Input: part model. Units: mm. Frame: model coordinates. Face numbers are marked on the shaded views. A direction names the side the tool comes from. Give positions to 0.01 mm unless a question says otherwise; leave off trailing zeros. Order: outer loops, then holes, each group sorted by start corner. A loop starts at its lowest first (then second) coordinate and runs counter-clockwise, first axis right, second up. Notation, with made-up numbers: (-12, -39.75) - (47, -39.75) arc R20 ccw to (47, -0.75) - close; hole circle Ø8 at (-28.5, 28). An arc over 180 degrees is marked (long way). Answer in a Markdown table with one row per item. Add a question column.
from build123d import *

# Parameters (mm, degrees)
BOSS_EXTRUDE3_DEPTH      = 1.5875
BOSS_EXTRUDE3_DEPTH_BACK = 43.175
SKETCH4_W                = 26.136325312
SKETCH4_H                = 38.4125
CUT_EXTRUDE1_DEPTH       = 14.701439982
SKETCH5_W                = 2
SKETCH5_H                = 2
BOSS_EXTRUDE5_DEPTH      = 44.7625
BOSS_EXTRUDE6_START      = -41.5875
SKETCH5_4_W              = 2
SKETCH5_4_H              = 2
BOSS_EXTRUDE6_DEPTH      = 38.4125


with BuildPart() as part:
    # Sketch3 → Boss-Extrude3 (new, two sides: drawn at the far end of the back side and taken through both)
    with BuildSketch(Plane.XY.offset(336.564940884).offset(-BOSS_EXTRUDE3_DEPTH_BACK)):
        with BuildLine():
            Line((-13.068162656, -2.834098381), (13.068162656, -2.834098381))
            ThreePointArc((13.068162656, -2.834098381), (15.189482999, -1.955418725), (16.068162656, 0.165901619))
            Line((16.068162656, 0.165901619), (16.068162656, 13.867341601))
            ThreePointArc((16.068162656, 13.867341601), (15.189482999, 15.988661944), (13.068162656, 16.867341601))
            Line((13.068162656, 16.867341601), (-13.068162656, 16.867341601))
            ThreePointArc((-13.068162656, 16.867341601), (-15.189482999, 15.988661944), (-16.068162656, 13.867341601))
            Line((-16.068162656, 13.867341601), (-16.068162656, 0.165901619))
            ThreePointArc((-16.068162656, 0.165901619), (-15.189482999, -1.955418725), (-13.068162656, -2.834098381))
        make_face()
    extrude(amount=BOSS_EXTRUDE3_DEPTH + BOSS_EXTRUDE3_DEPTH_BACK)

    # Sketch4 → Cut-Extrude1 (cut)
    with BuildSketch(Plane(origin=(0, 16.867341601, 0), x_dir=(1, 0, 0), z_dir=(0, 1, 0))):
        with Locations((0, -315.771190884)):
            Rectangle(SKETCH4_W, SKETCH4_H)
    extrude(amount=-CUT_EXTRUDE1_DEPTH, mode=Mode.SUBTRACT)

    # Sketch5 → Boss-Extrude5 (add)
    with BuildSketch(Plane.XY.offset(338.152440884)):
        with Locations((-17.068162656, 5)):
            Rectangle(SKETCH5_W, SKETCH5_H)
        with Locations((17.068162656, 5)):
            Rectangle(SKETCH5_W, SKETCH5_H)
    extrude(amount=-BOSS_EXTRUDE5_DEPTH)

    # Sketch5<4> → Boss-Extrude6 (add)
    with BuildSketch(Plane.XY.offset(338.152440884).offset(BOSS_EXTRUDE6_START)):
        with Locations((19.068162656, 5)):
            Rectangle(SKETCH5_4_W, SKETCH5_4_H)
        with Locations((-19.068162656, 5)):
            Rectangle(SKETCH5_4_W, SKETCH5_4_H)
    extrude(amount=BOSS_EXTRUDE6_DEPTH)


solid = part.part
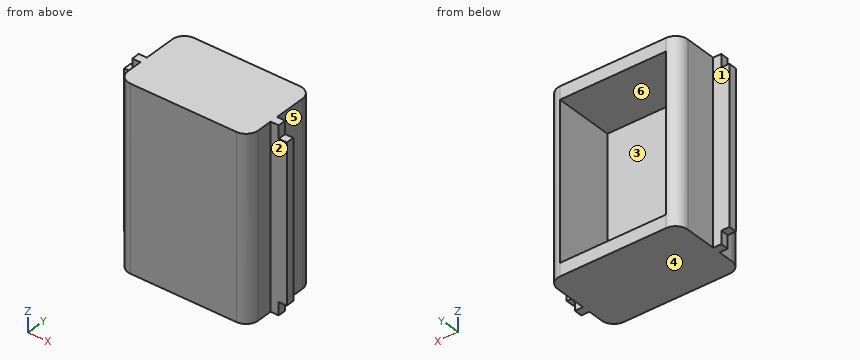
Q1. Section C-C, the plane x = 2. Return loops of the section in (y, z), then the cut area to 3 significant figures.
Q2. Contact query for flat-ended pins moving along their axis: P1, Ø2, axis at x = 19, y = 5.5, coming from the -Z side; P2, Ø1, axis at y = 7, z = 323, coming from the -X side; P3, Ø2, axis at y = 5, z = 294.5, coming from the -X side; P4, Ø5, axis at y = 13.5, z = 332, coming from the +X side. Output: stop coordinate, or through.
Q3. Line query: probe 1 along X at (y, z) = (12.25, 322.5); probe 2 along X at (y, z) = (5.75, 323.5); probe 3 along Z at (x, y) = (9, 5.5). Output: solid intervals per line, ascending.
Q4. Access query for the marked faces 1, 2 and 3. Directions: +Z, -Z, +X, -X, +Y, -Y. A direction counts if a zero-diameter tool reaches every point of the face in a straight line with its end or side. Return the directions, or none.
Q5. Section A-A, the plane y = 9.75. Return loops of the section in (x, z), then the cut area to 3 significant figures.
Q6. Pull-direction query (Z, two-part tool) for the marked faces 4, 5 and 6; classes: +Z half, -Z half, draft (parallel to the pull), parting line (faces both ways), or undercut.
Q7. Section B-B, the plane z = 331.5. Return loops of the section in (x, y).
Computed:
| question | item | result |
|---|---|---|
| 1 | outline | (-2.83, 293.39) - (16.87, 293.39) - (16.87, 296.56) - (2.17, 296.56) - (2.17, 334.98) - (16.87, 334.98) - (16.87, 338.15) - (-2.83, 338.15) - close |
| 1 | area | 317 mm^2 |
| 2 | P1 | stops at z = 293.39 |
| 2 | P2 | stops at x = -16.07 |
| 2 | P3 | stops at x = -18.07 |
| 2 | P4 | stops at x = 16.07 |
| 3 | probe 1 | x = -16.07 to -13.07, 13.07 to 16.07 |
| 3 | probe 2 | x = -20.07 to -13.07, 13.07 to 20.07 |
| 3 | probe 3 | z = 293.39 to 296.56, 334.98 to 338.15 |
| 4 | face 1 | +Z, -Z, -X, +Y |
| 4 | face 2 | +Z, -Z, +X, -Y |
| 4 | face 3 | +Y |
| 5 | outline | (-16.07, 293.39) - (16.07, 293.39) - (16.07, 338.15) - (-16.07, 338.15) - close; hole (-13.07, 296.56) - (13.07, 296.56) - (13.07, 334.98) - (-13.07, 334.98) - close |
| 5 | area | 435 mm^2 |
| 6 | face 4 | -Z half |
| 6 | face 5 | draft |
| 6 | face 6 | undercut |
| 7 | outline | (-20.07, 4) - (-16.07, 4) - (-16.07, 0.17) arc R3 ccw to (-13.07, -2.83) - (13.07, -2.83) arc R3 ccw to (16.07, 0.17) - (16.07, 4) - (20.07, 4) - (20.07, 6) - (16.07, 6) - (16.07, 13.87) arc R3 ccw to (13.07, 16.87) - (13.07, 2.17) - (-13.07, 2.17) - (-13.07, 16.87) arc R3 ccw to (-16.07, 13.87) - (-16.07, 6) - (-20.07, 6) - close |
